```python
from build123d import *

# Parameters (mm, degrees)
SKETCH1_W           = 70
SKETCH1_H           = 85
BOSS_EXTRUDE1_DEPTH = 2.5
SKETCH2_W           = 10.5
SKETCH2_H           = 60
CUT_EXTRUDE1_DEPTH  = 10
SKETCH3_W           = 2.519429159
SKETCH3_H           = 8
CUT_EXTRUDE2_DEPTH  = 10
SKETCH4_W           = 4.7
SKETCH4_H           = 4.7
SKETCH4_W_2         = 29.9
SKETCH4_H_2         = 7.6
CUT_EXTRUDE3_DEPTH  = 10
BOSS_EXTRUDE2_DEPTH = 13
SKETCH8_W           = 10
SKETCH8_H           = 1.2
CUT_EXTRUDE6_DEPTH  = 9.5
SKETCH9_R           = 6.15
CUT_EXTRUDE7_DEPTH  = 20
SKETCH10_W          = 10
SKETCH10_H          = 1.2
CUT_EXTRUDE8_DEPTH  = 9.5
SKETCH11_R          = 6.15
CUT_EXTRUDE9_DEPTH  = 20
CUT_EXTRUDE10_DEPTH = 1.2
SKETCH13_W          = 3
SKETCH13_H          = 4.191956584
CUT_EXTRUDE11_DEPTH = 1.2
SKETCH15_R          = 1.5
CUT_EXTRUDE12_DEPTH = 10
SKETCH16_R          = 2
CUT_EXTRUDE13_DEPTH = 10
SKETCH17_W          = 64.961141682
SKETCH17_H          = 2
BOSS_EXTRUDE3_DEPTH = 15.5
FILLET1_R           = 5
SKETCH18_W          = 7.984996169
SKETCH18_H          = 62.989999862
CUT_EXTRUDE14_DEPTH = 50
CUT_EXTRUDE15_DEPTH = 2


with BuildPart() as part:
    # Sketch1 → Boss-Extrude1 (new body)
    with BuildSketch(Plane(origin=(0, 0, 0), x_dir=(1, 0, 0), z_dir=(0, 1, 0))):
        Rectangle(SKETCH1_W, SKETCH1_H)
    extrude(amount=BOSS_EXTRUDE1_DEPTH)

    # Sketch2 → Cut-Extrude1 (cut)
    with BuildSketch(Plane(origin=(0, 0, 0), x_dir=(-1, 0, 0), z_dir=(0, -1, 0))):
        with Locations((-29.75, -4.5)):
            Rectangle(SKETCH2_W, SKETCH2_H)
        with Locations((29.75, -4.5)):
            Rectangle(SKETCH2_W, SKETCH2_H)
    extrude(amount=-CUT_EXTRUDE1_DEPTH, mode=Mode.SUBTRACT)

    # Sketch3 → Cut-Extrude2 (cut)
    with BuildSketch(Plane(origin=(0, 2.5, 0), x_dir=(1, 0, 0), z_dir=(0, 1, 0))):
        Polygon((17.462549034, 42.5), (35, 42.5), (35, 25.5), (32.484854108, 25.5), (32.484996169, 27.489999862), align=None)
        with Locations((33.740285421, -38.5)):
            Rectangle(SKETCH3_W, SKETCH3_H)
        with Locations((-33.740285421, -38.5)):
            Rectangle(SKETCH3_W, SKETCH3_H)
        Polygon((-32.484996169, 27.489999862), (-17.462549034, 42.5), (-35, 42.5), (-35, 25.5), (-32.484854108, 25.5), align=None)
    extrude(amount=-CUT_EXTRUDE2_DEPTH, mode=Mode.SUBTRACT)

    # Sketch4 → Cut-Extrude3 (cut)
    with BuildSketch(Plane(origin=(0, 0, 0), x_dir=(-1, 0, 0), z_dir=(0, -1, 0))):
        with Locations((-17, 3.5)):
            Rectangle(SKETCH4_W, SKETCH4_H)
        with Locations((-17, -12.5)):
            Rectangle(SKETCH4_W, SKETCH4_H)
        with Locations((17, -12.5)):
            Rectangle(SKETCH4_W, SKETCH4_H)
        with Locations((17, 3.5)):
            Rectangle(SKETCH4_W, SKETCH4_H)
        with Locations((0, 32.6)):
            Rectangle(SKETCH4_W_2, SKETCH4_H_2)
    extrude(amount=-CUT_EXTRUDE3_DEPTH, mode=Mode.SUBTRACT)

    # Sketch5 → Boss-Extrude2 (add)
    with BuildSketch(Plane(origin=(0, 2.5, 0), x_dir=(1, 0, 0), z_dir=(0, 1, 0))):
        Polygon((-32.484996169, 27.489999862), (-32.484854108, 25.5), (-24.5, 25.5), (-24.5, 22.7), (-18.8, 22.7), (-18.8, 25.8), (-15.2, 25.8), (-15.2, 22.7), (-8.5, 22.7), (-8.5, 28.8), (-15.962549034, 28.8), (-15.962549034, 30.4), (-19, 30.4), (-19, 32.5), (-15.962549034, 32.5), (-15.962549034, 42.5), (-17.462549034, 42.5), align=None)
        Polygon((-9.5, -42.5), (-9.5, -31.7), (-15.2, -31.7), (-15.2, -34.8), (-18.8, -34.8), (-18.8, -31.7), (-24.5, -31.7), (-24.5, -34.5), (-32.480570841, -34.5), (-32.480570841, -42.5), align=None)
        Polygon((32.480570841, -42.5), (9.5, -42.5), (9.5, -31.7), (15.2, -31.7), (15.2, -34.8), (18.8, -34.8), (18.8, -31.7), (24.5, -31.7), (24.5, -34.5), (32.480570841, -34.5), align=None)
        Polygon((15.962549034, 30.4), (15.962549034, 28.8), (8.5, 28.8), (8.5, 22.7), (15.2, 22.7), (15.2, 25.8), (18.8, 25.8), (18.8, 22.7), (24.5, 22.7), (24.5, 25.5), (32.484854108, 25.5), (32.484996169, 27.489999862), (17.462549034, 42.5), (15.962549034, 42.5), (15.962549034, 32.5), (19, 32.5), (19, 30.4), align=None)
    extrude(amount=BOSS_EXTRUDE2_DEPTH)

    # Sketch8 → Cut-Extrude6 (cut)
    with BuildSketch(Plane.ZY.offset(24.5)):
        with Locations((23.5, 1.9)):
            Rectangle(SKETCH8_W, SKETCH8_H)
    extrude(amount=-CUT_EXTRUDE6_DEPTH, mode=Mode.SUBTRACT)

    # Sketch9 → Cut-Extrude7 (cut)
    with BuildSketch(Plane.ZY.offset(15)):
        with Locations((23.5, 7)):
            Circle(SKETCH9_R)
    extrude(amount=-CUT_EXTRUDE7_DEPTH, mode=Mode.SUBTRACT)

    # Sketch10 → Cut-Extrude8 (cut)
    with BuildSketch(Plane(origin=(24.5, 0, 0), x_dir=(0, 0, -1), z_dir=(1, 0, 0))):
        with Locations((14.5, 1.9)):
            Rectangle(SKETCH10_W, SKETCH10_H)
    extrude(amount=-CUT_EXTRUDE8_DEPTH, mode=Mode.SUBTRACT)

    # Sketch11 → Cut-Extrude9 (cut)
    with BuildSketch(Plane(origin=(15, 0, 0), x_dir=(0, 0, -1), z_dir=(1, 0, 0))):
        with Locations((14.5, 7)):
            Circle(SKETCH11_R)
    extrude(amount=-CUT_EXTRUDE9_DEPTH, mode=Mode.SUBTRACT)

    # Sketch12 → Cut-Extrude10 (cut)
    with BuildSketch(Plane(origin=(0, 2.5, 0), x_dir=(1, 0, 0), z_dir=(0, 1, 0))):
        Polygon((5, -19.308043416), (7.5, -19.308043416), (7.5, 10.308043416), (-7.5, 10.308043416), (-7.5, -19.308043416), align=None)
    extrude(amount=-CUT_EXTRUDE10_DEPTH, mode=Mode.SUBTRACT)

    # Sketch13 → Cut-Extrude11 (cut)
    with BuildSketch(Plane(origin=(0, 2.5, 0), x_dir=(1, 0, 0), z_dir=(0, 1, 0))):
        with Locations((-0.8, 12.404021708)):
            Rectangle(SKETCH13_W, SKETCH13_H)
        with Locations((0.8, -21.404021708)):
            Rectangle(SKETCH13_W, SKETCH13_H)
    extrude(amount=-CUT_EXTRUDE11_DEPTH, mode=Mode.SUBTRACT)

    # Sketch15 → Cut-Extrude12 (cut)
    with BuildSketch(Plane(origin=(0, 2.5, 0), x_dir=(1, 0, 0), z_dir=(0, 1, 0))):
        with Locations(Location((0, 25, 0), (0, 0, 270))):
            Circle(SKETCH15_R)
        with Locations(Location((0, -40, 0), (0, 0, 270))):
            Circle(SKETCH15_R)
    extrude(amount=-CUT_EXTRUDE12_DEPTH, mode=Mode.SUBTRACT)

    # Sketch16 → Cut-Extrude13 (cut)
    with BuildSketch(Plane(origin=(0, 15.5, 0), x_dir=(1, 0, 0), z_dir=(0, 1, 0))):
        with Locations(Location((12.39, 25.4, 0), (0, 0, 270))):
            Circle(SKETCH16_R)
        with Locations(Location((17, -39, 0), (0, 0, 270))):
            Circle(SKETCH16_R)
        with Locations(Location((-17, -39, 0), (0, 0, 90))):
            Circle(SKETCH16_R)
        with Locations(Location((-12.39, 25.4, 0), (0, 0, 90))):
            Circle(SKETCH16_R)
    extrude(amount=-CUT_EXTRUDE13_DEPTH, mode=Mode.SUBTRACT)

    # Sketch17 → Boss-Extrude3 (add)
    with BuildSketch(Plane(origin=(0, 0, 0), x_dir=(-1, 0, 0), z_dir=(0, -1, 0))):
        with Locations((0, -43.5)):
            Rectangle(SKETCH17_W, SKETCH17_H)
    extrude(amount=-BOSS_EXTRUDE3_DEPTH)

    # Fillet1
    fillet1_edges = [part.edges().sort_by_distance(p)[0] for p in [
        (-32.480570841, 7.75, 44.5),
        (32.480570841, 7.75, 44.5),
    ]]
    fillet(fillet1_edges, radius=FILLET1_R)

    # Sketch18 → Cut-Extrude14 (cut, symmetric)
    with BuildSketch(Plane(origin=(0, 2.5, 0), x_dir=(1, 0, 0), z_dir=(0, 1, 0))):
        with Locations((-28.492498084, -4.005000069)):
            Rectangle(SKETCH18_W, SKETCH18_H)
        with Locations((28.492498084, -4.005000069)):
            Rectangle(SKETCH18_W, SKETCH18_H)
    extrude(amount=CUT_EXTRUDE14_DEPTH, both=True, mode=Mode.SUBTRACT)

    # Sketch19 → Cut-Extrude15 (cut)
    with BuildSketch(Plane(origin=(0, 2.5, 0), x_dir=(1, 0, 0), z_dir=(0, 1, 0))):
        Polygon((15, 18.691956584), (-5, 18.691956584), (-7.5, 18.691956584), (-7.5, -19.308043416), (-15, -19.308043416), (-15, -27.691956584), (5, -27.691956584), (5, -19.308043416), (7.5, -19.308043416), (7.5, 10.308043416), (15, 10.308043416), align=None)
    extrude(amount=-CUT_EXTRUDE15_DEPTH, mode=Mode.SUBTRACT)


solid = part.part
```
Read the model definition and answer for the solid it produces. Units are mm, in the model's axes. A direction names the side the tool comes from. Coordinates: 2 decimals unless noted, no trailing zeros. Loops run counter-clockwise (first coordinate to the right, second up) from the corner with the lowest first, then second, coordinate; pieces in that order, holes last. Notation, with made-up numbers: (-25.5, 17) -> (-10.5, 17) arc R23 ccw to (-10.5, 26) -> close; hole circle Ø1 at (32, 8). An arc over 180 degrees is marked (long way). Return JSON: item names as keys, results as strings.
Item 1: For faces 4 (the flat face through (-8.5, 9, -26)), 5 (the flat face through (-15.2, 9, -24)), 6 (the flat face through (28, 8, -27.49)), 7 (the flat face through (-19.35, 1, 13)), determine the directions among +Z, -Z, +X, -X, +Y, -Y from which every point of the face is accessible in a straight line to the end or side of a thin tool.
Answers:
{"face 4": "-Z, +Y", "face 5": "+Y", "face 6": "+X, +Y, -Y", "face 7": "+Y, -Y"}
Item 2: Find section A-A (x = -6). Determine the outline of the cut face in (y, z), plus the area to 3 significant figures.
Answers:
{"outline": "(0, -42.5) -> (2.5, -42.5) -> (2.5, -36.4) -> (0, -36.4) -> close; (0, -28.8) -> (2.5, -28.8) -> (2.5, -18.69) -> (0.5, -18.69) -> (0.5, 27.69) -> (2.5, 27.69) -> (2.5, 42.5) -> (15.5, 42.5) -> (15.5, 44.5) -> (0, 44.5) -> close", "area": "132 mm2"}
Item 3: Find section C-C (y = 10.5). Count the separate pieces of the cut face and the enclosed holes in it, plus the area to 3 significant figures.
Answers:
{"separate pieces": "3", "enclosed holes": "4", "area": "891 mm2"}
Item 4: Find section D-D (z = -7.5). Determine the outline of the cut face in (x, y).
Answers:
{"outline": "(-24.5, 0) -> (24.5, 0) -> (24.5, 2.5) -> (7.5, 2.5) -> (7.5, 0.5) -> (-7.5, 0.5) -> (-7.5, 2.5) -> (-24.5, 2.5) -> close"}
Item 5: Find section B-B (z = -34). Determine the outline of the cut face in (x, y), plus the area to 3 significant figures.
Answers:
{"outline": "(-25.97, 0) -> (-14.95, 0) -> (-14.95, 2.5) -> (-15.96, 2.5) -> (-15.96, 15.5) -> (-25.97, 15.5) -> close; (14.95, 0) -> (25.97, 0) -> (25.97, 15.5) -> (15.96, 15.5) -> (15.96, 2.5) -> (14.95, 2.5) -> close", "area": "315 mm2"}
Item 6: Flat-ended cylindrical pins translate along their axes: P1, Ø0.9, axis at y = 9, z = 33.5, coming from the -X side; P2, Ø4.5, axis at x = 18, z = 38.5, coming from the +Y side; P3, Ø3, axis at y = 2, z = -4, coming from the +X side; P4, Ø0.5, axis at y = 7.5, z = -29.5, coming from the +X side. Find the tip coordinate at first contact, or state that the pin passes through.
Answers:
{"P1": "stops at x = -24.5", "P2": "stops at y = 15.5", "P3": "stops at x = 24.5", "P4": "stops at x = 30.72"}
Item 7: Find the intervals of material crossed by probe 1 along Z at (x, y) = (-12.39, 9); probe 2 along Z at (x, y) = (-17, 11); probe 3 along X at (y, z) = (12.75, -25.4), in increasing order.
Answers:
{"probe 1": "z = -28.8 to -27.4, -23.4 to -22.7, 31.7 to 44.5", "probe 2": "z = -42.5 to -32.5, -30.4 to -25.8, 34.8 to 37, 41 to 44.5", "probe 3": "x = -24.5 to -18.8, -15.2 to -14.39, -10.39 to -8.5, 8.5 to 10.39, 14.39 to 15.2, 18.8 to 24.5"}
Item 8: For a pull along Z with two mould halves and no side action, classify faces 1 (the flat face through (18.8, 9, -24)), 2 (the flat face through (15.2, 9, -24)), 3 (the flat face through (15.963, 9, -38)) as +Z half, -Z half, draft (parallel to the pull), parting line (faces both ways), or undercut.
Answers:
{"face 1": "undercut", "face 2": "undercut", "face 3": "draft"}
